The model under review builds one solid part; all positions refer to its coordinate system, in mm. A direction names the side the tool comes from. Coordinates: 2 decimals unless noted, no trailing zeros. Write each loop counter-clockwise with the first axis right and the second up, starting at its lowest first coordinate (ties: lowest second). Pieces come first, ordered by that corner, then holes.
```python
from build123d import *

# Parameters (mm, degrees)
BOSS_EXTRUDE1_DEPTH = 12.7
SKETCH2_R           = 7.9375
CUT_EXTRUDE1_DEPTH  = 25.4
CUT_EXTRUDE2_DEPTH  = 15.24
CUT_EXTRUDE4_DEPTH  = 12.7
CUT_EXTRUDE3_DEPTH  = 12.7
FILLET4_R           = 3.81
CUT_EXTRUDE8_REACH  = 306.459
SKETCH10_R          = 3.302
CUT_EXTRUDE11_DEPTH = 12.7
BOSS_EXTRUDE2_DEPTH = 12.7


with BuildPart() as part:
    # Sketch1 → Boss-Extrude1 (new body)
    with BuildSketch(Plane.XY):
        with BuildLine():
            Line((22.605250022, 67.052290313), (98.805250022, 67.052290313))
            Line((98.805250022, 67.052290313), (98.805250022, 155.952290313))
            Line((98.805250022, 155.952290313), (-49.161223166, 287.699993186))
            ThreePointArc((-49.161223166, 287.699993186), (-96.236474745, 204.218681994), (-40.152034083, 126.502891159))
            Line((-40.152034083, 126.502891159), (22.605250022, 130.274128502))
            Line((22.605250022, 130.274128502), (22.605250022, 67.052290313))
        make_face()
    extrude(amount=BOSS_EXTRUDE1_DEPTH)

    # Sketch2 → Cut-Extrude1 (cut)
    with BuildSketch(Plane.XY.offset(12.7)):
        with Locations((-7.239749978, 209.038290313)):
            Circle(SKETCH2_R)
    extrude(amount=-CUT_EXTRUDE1_DEPTH, mode=Mode.SUBTRACT)

    # Sketch3 → Cut-Extrude2 (cut)
    with BuildSketch(Plane.XY.offset(12.7)):
        Polygon((41.655250022, 70.862290313), (41.655250022, 83.562290313), (60.705250022, 108.644790313), (79.755250022, 83.562290313), (79.755250022, 70.862290313), align=None)
        Polygon((26.415250022, 86.102290313), (39.115250022, 86.102290313), (57.847750022, 111.502290313), (39.115250022, 136.902290313), (26.415250022, 136.902290313), align=None)
        Polygon((94.995250022, 86.102290313), (82.295250022, 86.102290313), (63.562750022, 111.502290313), (82.295250022, 136.902290313), (94.995250022, 136.902290313), align=None)
        Polygon((41.655250022, 152.142290313), (41.655250022, 139.442290313), (60.705250022, 114.359790313), (79.755250022, 139.442290313), (79.755250022, 152.142290313), align=None)
    extrude(amount=-CUT_EXTRUDE2_DEPTH, mode=Mode.SUBTRACT)

    # Sketch5 → Cut-Extrude4 (cut)
    with BuildSketch(Plane.XY.offset(12.7)):
        with BuildLine():
            Line((-0.75941726, 237.80168728), (-42.818220106, 275.250377791))
            ThreePointArc((-42.818220106, 275.250377791), (-81.480920705, 220.910985735), (-61.519248594, 157.278402939))
            Line((-61.519248594, 157.278402939), (-20.395339746, 203.464861019))
            ThreePointArc((-20.395339746, 203.464861019), (-21.336998363, 211.362132865), (-17.910409102, 218.539326578))
            Line((-17.910409102, 218.539326578), (-0.75941726, 237.80168728))
        make_face()
        Polygon((-36.620175939, 130.532002023), (-56.03788631, 155.851799386), (-20.994230128, 195.20949671), (20.700250022, 172.076525379), (20.700250022, 133.976525379), align=None)
        with BuildLine():
            Line((-5.26797782, 223.189077245), (3.983097906, 233.579004496))
            Line((3.983097906, 233.579004496), (15.365134305, 223.444565813))
            Line((15.365134305, 223.444565813), (6.380422315, 213.353792944))
            ThreePointArc((6.380422315, 213.353792944), (1.977645927, 219.954895508), (-5.26797782, 223.189077245))
        make_face()
    extrude(amount=-CUT_EXTRUDE4_DEPTH, mode=Mode.SUBTRACT)

    # Sketch4 → Cut-Extrude3 (cut)
    with BuildSketch(Plane.XY.offset(12.7)):
        Polygon((57.615510223, 155.952290313), (-5.197073481, 190.802028044), (20.952186028, 220.170386062), (68.306030681, 178.007049188), (68.306030681, 155.952290313), align=None)
        Polygon((91.166030681, 155.952290313), (70.846030681, 155.952290313), (70.846030681, 174.044992428), align=None)
    extrude(amount=-CUT_EXTRUDE3_DEPTH, mode=Mode.SUBTRACT)

    # Fillet4
    fillet4_edges = [part.edges().sort_by_distance(p)[0] for p in [
        (-20.994230128, 195.20949671, 6.35),
        (57.615510223, 155.952290313, 6.35),
    ]]
    fillet(fillet4_edges, radius=FILLET4_R)

    # Sketch10 → Cut-Extrude8 (cut, up to next)
    with BuildSketch(Plane.XY.offset(12.7), mode=Mode.PRIVATE) as cut_extrude8_sk1:
        with Locations((32.765250022, 77.212290313)):
            Circle(SKETCH10_R)
    cut_extrude8_tool1 = extrude(cut_extrude8_sk1.sketch, amount=-CUT_EXTRUDE8_REACH, mode=Mode.PRIVATE) & part.part
    # Sketch10 → Cut-Extrude8 (cut, up to next)
    with BuildSketch(Plane.XY.offset(12.7), mode=Mode.PRIVATE) as cut_extrude8_sk2:
        with Locations((32.765250022, 145.792290313)):
            Circle(SKETCH10_R)
    cut_extrude8_tool2 = extrude(cut_extrude8_sk2.sketch, amount=-CUT_EXTRUDE8_REACH, mode=Mode.PRIVATE) & part.part
    # Sketch10 → Cut-Extrude8 (cut, up to next)
    with BuildSketch(Plane.XY.offset(12.7), mode=Mode.PRIVATE) as cut_extrude8_sk3:
        with Locations((88.645250022, 145.792290313)):
            Circle(SKETCH10_R)
    cut_extrude8_tool3 = extrude(cut_extrude8_sk3.sketch, amount=-CUT_EXTRUDE8_REACH, mode=Mode.PRIVATE) & part.part
    # Sketch10 → Cut-Extrude8 (cut, up to next)
    with BuildSketch(Plane.XY.offset(12.7), mode=Mode.PRIVATE) as cut_extrude8_sk4:
        with Locations((88.645250022, 77.212290313)):
            Circle(SKETCH10_R)
    cut_extrude8_tool4 = extrude(cut_extrude8_sk4.sketch, amount=-CUT_EXTRUDE8_REACH, mode=Mode.PRIVATE) & part.part
    add(cut_extrude8_tool1.solids().sort_by_distance((32.76525, 77.21229, 12.7))[0], mode=Mode.SUBTRACT)
    add(cut_extrude8_tool2.solids().sort_by_distance((32.76525, 145.79229, 12.7))[0], mode=Mode.SUBTRACT)
    add(cut_extrude8_tool3.solids().sort_by_distance((88.64525, 145.79229, 12.7))[0], mode=Mode.SUBTRACT)
    add(cut_extrude8_tool4.solids().sort_by_distance((88.64525, 77.21229, 12.7))[0], mode=Mode.SUBTRACT)

    # Sketch14 → Cut-Extrude11 (cut)
    with BuildSketch(Plane.XY.offset(12.7)):
        Polygon((-0.75941726, 237.80168728), (-90.284904, 256.297301642), (-56.503441725, 294.237422972), (2.618728967, 241.595699413), align=None)
    extrude(amount=-CUT_EXTRUDE11_DEPTH, mode=Mode.SUBTRACT)

    # Sketch15 → Boss-Extrude2 (add)
    with BuildSketch(Plane.XY.offset(12.7)):
        Polygon((2.618728967, 241.595699413), (-83.695447283, 254.935945734), (-84.471371658, 249.915553183), (-1.404499457, 237.07719239), align=None)
    extrude(amount=-BOSS_EXTRUDE2_DEPTH)


solid = part.part
```
Item 1: For pin 1 (6.5 mm diameter, centred on y = 100, z = 7.5, fed in from -X); pin 2 (10.5 mm diameter, centred on x = 88.65, y = 77.21, fed in from -Z); pin 3 (3 mm diameter, centred on y = 182.5, z = 2.5, fed in from -X); pin 4 (4 mm diameter, centred on y = 178.5, z = 9, fed in from +X), all flat-tipped, find the tip position at first contact; note any pin that passes through.
Solved:
pin 1: stops at x = 22.61
pin 2: stops at z = 0
pin 3: stops at x = -92.73
pin 4: stops at x = 75.73
Item 2: Take a section at D-D, the plane x = 18. Write out the cut boundary in (y, z).
Solved:
outline: (130, 0) - (133.81, 0) - (133.81, 12.7) - (130, 12.7) - close; (173.57, 0) - (177.93, 0) - (177.93, 12.7) - (173.57, 12.7) - close; (216.85, 0) - (227.9, 0) - (227.9, 12.7) - (216.85, 12.7) - close
Item 3: To check wall thickness, follow line 1 along X through (y, z) = (111.5, 10.5); line 2 along X through (y, z) = (166, 11.5); line 3 along Y through (x, z) = (-50, 9.25). State the ranges of each line that lie inside material, in increasing order.
Solved:
line 1: x = 22.61 to 26.42, 57.85 to 63.56, 95 to 98.81
line 2: x = -85.18 to -68.71, -53.75 to -47, 20.7 to 39.51, 68.31 to 70.85, 79.88 to 87.52
line 3: y = 131.11 to 147.98, 162.63 to 170.22, 244.59 to 249.73
Item 4: Take a section at B-B, the plane x = -75. Write out the cut boundary in (y, z), plus the area to 3 significant figures.
Solved:
outline: (151.36, 0) - (176.7, 0) - (176.7, 12.7) - (151.36, 12.7) - close; (241.66, 0) - (253.59, 0) - (253.59, 12.7) - (241.66, 12.7) - close
area: 473 mm2
Item 5: Take a section at A-A, the plane y = 186. Write out the cut boundary in (x, z), plus the area to 3 significant figures.
Solved:
outline: (-93.3, 0) - (-78.73, 0) - (-78.73, 12.7) - (-93.3, 12.7) - close; (-35.95, 0) - (-29.19, 0) - (-29.19, 12.7) - (-35.95, 12.7) - close; (-4.4, 0) - (3.46, 0) - (3.46, 12.7) - (-4.4, 12.7) - close; (59.33, 0) - (65.06, 0) - (65.06, 12.7) - (59.33, 12.7) - close
area: 443 mm2
Item 6: Take a section at C-C, the plane y = 230. Write out the cut boundary in (x, z), plus the area to 3 significant figures.
Solved:
outline: (-93.9, 0) - (-79.45, 0) - (-79.45, 12.7) - (-93.9, 12.7) - close; (-7.71, 0) - (0.8, 0) - (0.8, 12.7) - (-7.71, 12.7) - close; (8, 0) - (15.64, 0) - (15.64, 12.7) - (8, 12.7) - close
area: 388 mm2
Item 7: Machinability: for faces 1 (the face through (98.805, 111, 6)), 2 (the face through (-41.245, 180.048, 6.439)), which of the approach directions +Z, -Z, +X, -X, +Y, -Y give a long, thin tool a straight path to every point of the face, cutting with its end or side? Answer none if there is none.
Solved:
face 1: +Z, -Z, +X, +Y, -Y
face 2: +Z, -Z
Item 8: Mouldability with a two-part tool opening along Y and no side actions: class faces 3 (the face through (8, 182, 0)), 4 (the face through (-39.93, 248.17, 6.44)), 5 (the face through (80.86, 165.13, 6.44)) as pulls with the +Y half, pulls with the -Y half, needs draft (parallel to the pull), parting line crosses it, or undercut.
Solved:
face 3: needs draft
face 4: pulls with the +Y half
face 5: undercut
